Here's how the part is built. I have some questions about the finished solid (model axes, mm). Face numbers are marked on the shaded views. A direction names the side the tool comes from. Round coordinates to 2 decimals unless told otherwise and drop trailing zeros. Write each loop counter-clockwise with the first axis right and the second up, starting at its lowest first coordinate (ties: lowest second). Pieces come first, ordered by that corner, then holes. Notation, with made-up numbers: (80.25, 63) -> (93.25, 63) arc R17 ccw to (93.25, 83) -> close; hole circle Ø8 at (62.5, 8.25). An arc over 180 degrees is marked (long way). Put each result on its own line as item: value. Start each with the question number.
1) I want a section at A-A, the plane z = 16. List the corners of the cut face in (x, y) for me, then the cut area to 3 significant figures.
2) I want a section at D-D, the plane x = 5.5. List the corners of the cut face in (y, z) for me.
3) I want a section at C-C, the plane z = -10.5. List the corners of the cut face in (x, y) for me.
4) If I drill on line 1 along Z through (x, y) = (-11, 7.25); line 2 along Z through (x, y) = (-13.5, 6.25); line 3 along X through (y, z) = (10, 8), over which ranges is the centre line in solid material (lowest first)? Write a range as [from, to].
5) We'd pull the mould along X, two halves only. Please class the marked faces 4, 5, 6 and 7: released by +X, released by -X, zero draft, split by the parting line, or undercut.
6) Will these pins go through, and if not, where does the flat tip stop? P1, Ø8, axis at x = -5.5, y = 8.5, coming from the +Z side; P2, Ø1, axis at y = 3, z = -12, coming from the -X side; P3, Ø1.5, axis at y = 3.5, z = -3.5, coming from the -X side (3 decimals).
7) I want a section at B-B, the plane x = 14. List the corners of the cut face in (y, z) for me.
8) Which directions (+Z, -Z, +X, -X, +Y, -Y) give clear straight access to the entire face, cutting with the end or side of a thin tool? Please do the marked faces 1, 2 and 3.
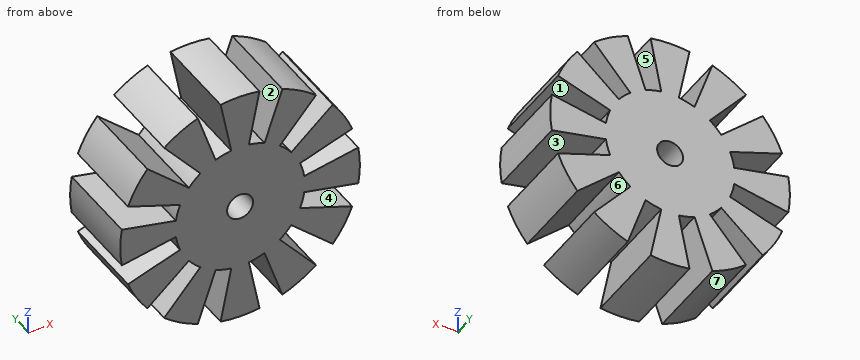
from build123d import *

# Parameters (mm, degrees)
SKETCH1_R           = 2
BOSS_EXTRUDE1_DEPTH = 13.5


with BuildPart() as part:
    # Sketch1 → Boss-Extrude1 (new body)
    with BuildSketch(Plane(origin=(0, 0, 0), x_dir=(1, 0, 0), z_dir=(0, 1, 0))):
        with BuildLine():
            Line((-16.314190392, -6.686200591), (-8.263943043, -3.933992685))
            ThreePointArc((-8.263943043, -3.933992685), (-8.664036901, -2.744899122), (-8.912092237, -1.51506696))
            Line((-8.912092237, -1.51506696), (-17.259914901, -3.156708671))
            ThreePointArc((-17.259914901, -3.156708671), (-17.504778638, -0.156708671), (-17.259914901, 2.843291329))
            Line((-17.259914901, 2.843291329), (-8.912092237, 1.201649618))
            ThreePointArc((-8.912092237, 1.201649618), (-8.664036901, 2.43148178), (-8.263943043, 3.620575343))
            Line((-8.263943043, 3.620575343), (-16.314190392, 6.372783249))
            ThreePointArc((-16.314190392, 6.372783249), (-15.026248608, 9.093291329), (-13.314190392, 11.568935672))
            Line((-13.314190392, 11.568935672), (-6.905584753, 5.973320915))
            ThreePointArc((-6.905584753, 5.973320915), (-6.07584645, 6.914359141), (-5.134808223, 7.744097445))
            Line((-5.134808223, 7.744097445), (-10.730422981, 14.152703083))
            ThreePointArc((-10.730422981, 14.152703083), (-8.254778638, 15.864761299), (-5.534270558, 17.152703083))
            Line((-5.534270558, 17.152703083), (-2.782062651, 9.102455734))
            ThreePointArc((-2.782062651, 9.102455734), (-1.592969089, 9.502549592), (-0.363136927, 9.750604929))
            Line((-0.363136927, 9.750604929), (-2.004778638, 18.098427593))
            ThreePointArc((-2.004778638, 18.098427593), (0.995221362, 18.343291329), (3.995221362, 18.098427593))
            Line((3.995221362, 18.098427593), (2.353579652, 9.750604929))
            ThreePointArc((2.353579652, 9.750604929), (3.583411813, 9.502549592), (4.772505376, 9.102455734))
            Line((4.772505376, 9.102455734), (7.524713283, 17.152703083))
            ThreePointArc((7.524713283, 17.152703083), (10.245221362, 15.864761299), (12.720865705, 14.152703083))
            Line((12.720865705, 14.152703083), (7.125250948, 7.744097445))
            ThreePointArc((7.125250948, 7.744097445), (8.066289174, 6.914359141), (8.896027478, 5.973320915))
            Line((8.896027478, 5.973320915), (15.304633116, 11.568935672))
            ThreePointArc((15.304633116, 11.568935672), (17.016691332, 9.093291329), (18.304633116, 6.372783249))
            Line((18.304633116, 6.372783249), (10.254385767, 3.620575343))
            ThreePointArc((10.254385767, 3.620575343), (10.654479625, 2.43148178), (10.902534962, 1.201649618))
            Line((10.902534962, 1.201649618), (19.250357626, 2.843291329))
            ThreePointArc((19.250357626, 2.843291329), (19.495221362, -0.156708671), (19.250357626, -3.156708671))
            Line((19.250357626, -3.156708671), (10.902534962, -1.51506696))
            ThreePointArc((10.902534962, -1.51506696), (10.654479625, -2.744899122), (10.254385767, -3.933992685))
            Line((10.254385767, -3.933992685), (18.304633116, -6.686200591))
            ThreePointArc((18.304633116, -6.686200591), (17.016691332, -9.406708671), (15.304633116, -11.882353014))
            Line((15.304633116, -11.882353014), (8.896027478, -6.286738257))
            ThreePointArc((8.896027478, -6.286738257), (8.066289174, -7.227776483), (7.125250948, -8.057514787))
            Line((7.125250948, -8.057514787), (12.720865705, -14.466120425))
            ThreePointArc((12.720865705, -14.466120425), (10.245221362, -16.178178641), (7.524713283, -17.466120425))
            Line((7.524713283, -17.466120425), (4.772505376, -9.415873076))
            ThreePointArc((4.772505376, -9.415873076), (3.583411813, -9.815966934), (2.353579652, -10.06402227))
            Line((2.353579652, -10.06402227), (3.995221362, -18.411844934))
            ThreePointArc((3.995221362, -18.411844934), (0.995221362, -18.656708671), (-2.004778638, -18.411844934))
            Line((-2.004778638, -18.411844934), (-0.363136927, -10.06402227))
            ThreePointArc((-0.363136927, -10.06402227), (-1.592969089, -9.815966934), (-2.782062651, -9.415873076))
            Line((-2.782062651, -9.415873076), (-5.534270558, -17.466120425))
            ThreePointArc((-5.534270558, -17.466120425), (-8.254778638, -16.178178641), (-10.730422981, -14.466120425))
            Line((-10.730422981, -14.466120425), (-5.134808223, -8.057514787))
            ThreePointArc((-5.134808223, -8.057514787), (-6.07584645, -7.227776483), (-6.905584753, -6.286738257))
            Line((-6.905584753, -6.286738257), (-13.314190392, -11.882353014))
            ThreePointArc((-13.314190392, -11.882353014), (-15.026248608, -9.406708671), (-16.314190392, -6.686200591))
        make_face()
        with Locations(Location((0.995221362, -0.156708671, 0), (0, 0, 270))):
            Circle(SKETCH1_R, mode=Mode.SUBTRACT)
    extrude(amount=BOSS_EXTRUDE1_DEPTH)


solid = part.part
Findings:
1. outline: (-8.56, 0) -> (-5.03, 0) -> (-5.03, 13.5) -> (-8.56, 13.5) -> close; (-1.53, 0) -> (3.52, 0) -> (3.52, 13.5) -> (-1.53, 13.5) -> close; (7.02, 0) -> (10.55, 0) -> (10.55, 13.5) -> (7.02, 13.5) -> close
1. area: 163 mm2
2. outline: (0, -11.23) -> (13.5, -11.23) -> (13.5, 11.54) -> (0, 11.54) -> close
3. outline: (-14.13, 0) -> (-12.09, 0) -> (-12.09, 13.5) -> (-14.13, 13.5) -> close; (-7.54, 0) -> (-3.26, 0) -> (-3.26, 13.5) -> (-7.54, 13.5) -> close; (-0.51, 0) -> (2.5, 0) -> (2.5, 13.5) -> (-0.51, 13.5) -> close; (5.25, 0) -> (9.53, 0) -> (9.53, 13.5) -> (5.25, 13.5) -> close; (14.08, 0) -> (16.12, 0) -> (16.12, 13.5) -> (14.08, 13.5) -> close
4. line 1: z = [-9.55, -4.56], [-1.61, 1.93], [4.87, 9.86]
4. line 2: z = [-11.34, -5.41], [-2.1, 2.42], [5.72, 11.65]
4. line 3: x = [-15.76, -8.87], [-5.21, 7.2], [10.86, 17.75]
5. face 4: released by +X
5. face 5: undercut
5. face 6: undercut
5. face 7: released by -X
6. P1: stops at z = 18.49
6. P2: stops at x = -13.37
6. P3: stops at x = -17.275
7. outline: (0, -10.43) -> (13.5, -10.43) -> (13.5, -4.9) -> (0, -4.9) -> close; (0, -1.81) -> (13.5, -1.81) -> (13.5, 2.12) -> (0, 2.12) -> close; (0, 5.21) -> (13.5, 5.21) -> (13.5, 10.74) -> (0, 10.74) -> close
8. face 1: +X, +Y, -Y
8. face 2: +Z, +Y, -Y
8. face 3: +Y, -Y
